Here's how the part is built. I have some questions about the finished solid (model axes, mm). Face numbers are marked on the shaded views. Round coordinates to 2 decimals unless told otherwise and drop trailing zeros. Write each loop counter-clockwise with the first axis right and the second up, starting at its lowest first coordinate (ties: lowest second). Pieces come first, ordered by that corner, then holes. Notation, with made-up numbers: (13, 11) - (48, 11) arc R32 ccw to (48, 46) - close; hole circle Ø11 at (-31.75, 81). An arc over 180 degrees is marked (long way). One line per item, written item: value. Start each with the question number.
Item 1: For P1, Ø1.5, axis at y = 27, z = 3.5, coming from the -X side; P2, Ø1, axis at x = 22, y = 36, coming from the +Z side; P3, Ø0.8, axis at x = 32, z = 3.5, coming from the -Y side; P4, Ø4, axis at x = 20, y = 26, coming from the -Z side, each with a flat end and sliding along its axis, tell me the tip position at first contact or that it passes through.
Item 2: Imagine slicing it at B-B, the plane z = 2.75. Please give me the cut outline in (x, y).
Item 3: Thinking about a two-plate mould opening in Y: for the marked faces 1, 2 and 3, which applies, released by +Y, released by -Y, zero draft, split by the parting line, or undercut?
Item 4: Imagine slicing it at A-A, the plane y = 45. Please give me the cut outline in (x, z).
Item 5: If I drill on line 1 (Y direction, x = 29.75, z = 3.7); line 2 (X direction, y = 67.5, z = 3.9); line 3 (Z direction, x = 29, y = 61.5), over which ranges is the centre line in solid material (lowest first)?
Autodesk Fusion 360 part; units mm, degrees
sketch "Boceto1" plane through (0, 0, 0) normal (0, 0, 1) x (1, 0, 0)
  line L0 (37.3693, 70) -> (37.3693, 30.5735)
  line L1 (15.2693, 30.5734) -> (15.2693, 69.9734)
  arc A0 (15.2693, 30.5734) -> (37.3693, 30.5735) centre (26.3193, 30.5735) ccw
  arc A1 (37.3693, 70) -> (15.2693, 69.9734) centre (26.3193, 70) ccw
  line L2 (20.3193, 24.17) -> (20.3193, 34.5)
  line L3 (20.3193, 34.5) -> (32.3193, 34.5)
  line L4 (32.3193, 34.5) -> (32.3193, 24.17)
  line L5 (32.3193, 24.17) -> (31.3193, 24.17)
  line L6 (31.3193, 24.17) -> (31.3193, 33.5)
  line L7 (31.3193, 33.5) -> (21.3193, 33.5)
  line L8 (21.3193, 33.5) -> (21.3193, 24.17)
  line L9 (21.3193, 24.17) -> (20.3193, 24.17)
  line L10 (15.2693, 30.5734) -> (15.2693, 50.2734)
  line L11 (20.2878, 76.3829) -> (20.3003, 66.0529)
  line L12 (20.3003, 66.0529) -> (32.3002, 66.0673)
  line L13 (32.3002, 66.0673) -> (32.2878, 76.3973)
  line L14 (32.2878, 76.3973) -> (31.2878, 76.3961)
  line L15 (31.2878, 76.3961) -> (31.299, 67.0661)
  line L16 (31.299, 67.0661) -> (21.2991, 67.0541)
  line L17 (21.2991, 67.0541) -> (21.2878, 76.3841)
  line L18 (21.2878, 76.3841) -> (20.2878, 76.3829)
  dimension "d1" = 39.4
  dimension "d2" = 22.1
  dimension "d11" = 1
  dimension "d12" = 1
  dimension "d13" = 10
  dimension "d14" = 12
  dimension "d15" = 10.33
  dimension "d16" = 1
  dimension "d25" = 10.33
extrude "Extruir2" add sketch "Boceto1" along normal blind 5 contours L11 L12 L13 L14 L15 L16 L17 L18 makes body 1
extrude "Extruir3" add sketch "Boceto1" along normal blind 5 separate body contours L2 L3 L4 L5 L6 L7 L8 L9 makes body 2
extrude "Extruir4" add sketch "Boceto1" along normal blind 2 bodies 1 2
fillet "Empalme2" radius 1.9 5 edges at (26.3003, 66.0601, 2) (15.2693, 50.2734, 0) (26.3193, 19.5235, 0) (37.3693, 50.2867, 0) (26.306, 81.05, 0) on bodies 1
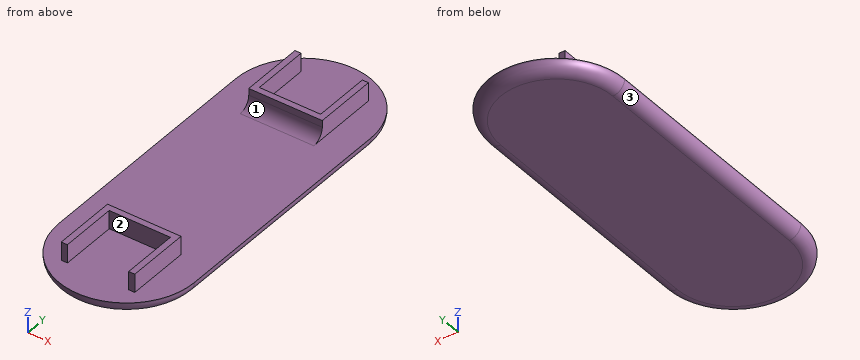
Values follow:
1. P1: stops at x = 20.32
1. P2: stops at z = 2
1. P3: stops at y = 24.17
1. P4: stops at z = 0
2. outline: (20.29, 76.38) - (20.3, 65.67) - (32.3, 65.68) - (32.29, 76.4) - (31.29, 76.4) - (31.3, 67.07) - (21.3, 67.05) - (21.29, 76.38) - close; (20.32, 24.17) - (21.32, 24.17) - (21.32, 33.5) - (31.32, 33.5) - (31.32, 24.17) - (32.32, 24.17) - (32.32, 34.5) - (20.32, 34.5) - close
3. face 1: undercut
3. face 2: released by -Y
3. face 3: zero draft
4. outline: (15.27, 1.9) arc R1.9 ccw to (17.17, 0) - (35.47, 0) arc R1.9 ccw to (37.37, 1.9) - (37.37, 2) - (15.27, 2) - close
5. line 1: y = 33.5 to 34.5, 66.05 to 67.06
5. line 2: x = 20.3 to 21.3, 31.3 to 32.3
5. line 3: z = 0 to 2
